Verification items for the finished model (mm, model axes). A direction names the side the tool comes from. Coordinates: 2 decimals unless noted, no trailing zeros. Write each loop counter-clockwise with the first axis right and the second up, starting at its lowest first coordinate (ties: lowest second). Pieces come first, ordered by that corner, then holes. Notation, with made-up numbers: M 12,30 L 42,30 A7 cw 42,40 Z; hole C 43.5,70 d4. An arc over 180 degrees is marked long. Answer in a Markdown table with one row per item.
from build123d import *

# Parameters (mm, degrees)
SKETCH_1_R          = 18
EXTRUDE_1_DEPTH     = 18.5
SKETCH_2_R          = 3
EXTRUDE_2_DEPTH     = 20
SKETCH_3_R          = 11
EXTRUDE_3_DEPTH     = 2
SKETCH_4_R          = 1.5
CUT_EXTRUDE_1_DEPTH = 8
SKETCH_5_R          = 4
EXTRUDE_4_DEPTH     = 20
EXTRUDE_START       = 2
SKETCH_6_R          = 11
EXTRUDE_5_DEPTH     = 2
CUT_EXTRUDE_START   = -8
SKETCH_7_R          = 1.5
CUT_EXTRUDE_2_DEPTH = 8
CUT_EXTRUDE_START_2 = -15
CUT_EXTRUDE_3_DEPTH = 15
CUT_EXTRUDE_4_DEPTH = 15
CHAMFER_1_SIZE      = 0.3


with BuildPart() as part:
    # 草图1 → 凸台-拉伸1 (new, symmetric)
    with BuildSketch(Plane.XY):
        Circle(SKETCH_1_R)
    extrude(amount=EXTRUDE_1_DEPTH, both=True)

    # 草图2 → 凸台-拉伸2 (add)
    with BuildSketch(Plane.XY.offset(18.5)):
        Circle(SKETCH_2_R)
    extrude(amount=EXTRUDE_2_DEPTH)

    # 草图3 → 凸台-拉伸3 (add)
    with BuildSketch(Plane.XY.offset(18.5)):
        Circle(SKETCH_3_R)
    extrude(amount=EXTRUDE_3_DEPTH)

    # 草图4 → 切除-拉伸1 (cut)
    with BuildSketch(Plane.XY.offset(18.5)):
        with Locations((-9.899494937, 9.899494937)):
            Circle(SKETCH_4_R)
        with Locations((9.899494937, 9.899494937)):
            Circle(SKETCH_4_R)
        with Locations((9.899494937, -9.899494937)):
            Circle(SKETCH_4_R)
        with Locations((-9.899494937, -9.899494937)):
            Circle(SKETCH_4_R)
    extrude(amount=-CUT_EXTRUDE_1_DEPTH, mode=Mode.SUBTRACT)

    # 草图5 → 凸台-拉伸4 (add)
    with BuildSketch(Plane(origin=(0, 0, -18.5), x_dir=(-1, 0, 0), z_dir=(0, 0, -1))):
        Circle(SKETCH_5_R)
    extrude(amount=EXTRUDE_4_DEPTH)

    # 草图6 → 凸台-拉伸5 (add)
    with BuildSketch(Plane(origin=(0, 0, -18.5), x_dir=(-1, 0, 0), z_dir=(0, 0, -1)).offset(EXTRUDE_START)):
        with Locations(Location((0, 0, 0), (0, 0, 180))):
            Circle(SKETCH_6_R)
    extrude(amount=-EXTRUDE_5_DEPTH)

    # 草图7 → 切除-拉伸2 (cut)
    with BuildSketch(Plane(origin=(0, 0, -18.5), x_dir=(-1, 0, 0), z_dir=(0, 0, -1)).offset(CUT_EXTRUDE_START)):
        with Locations(Location((-9.899494937, 9.899494937, 0), (0, 0, 180))):
            Circle(SKETCH_7_R)
        with Locations(Location((9.899494937, 9.899494937, 0), (0, 0, 180))):
            Circle(SKETCH_7_R)
        with Locations(Location((9.899494937, -9.899494937, 0), (0, 0, 180))):
            Circle(SKETCH_7_R)
        with Locations(Location((-9.899494937, -9.899494937, 0), (0, 0, 180))):
            Circle(SKETCH_7_R)
    extrude(amount=CUT_EXTRUDE_2_DEPTH, mode=Mode.SUBTRACT)

    # 草图8 → 切除-拉伸3 (cut)
    with BuildSketch(Plane.XY.offset(38.5).offset(CUT_EXTRUDE_START_2)):
        with BuildLine():
            Line((-2, 2.236067977), (-2, -2.236067977))
            ThreePointArc((-2, -2.236067977), (-3, 0), (-2, 2.236067977))
        make_face()
    extrude(amount=CUT_EXTRUDE_3_DEPTH, mode=Mode.SUBTRACT)

    # 草图9 → 切除-拉伸4 (cut)
    with BuildSketch(Plane(origin=(0, 0, -38.5), x_dir=(-1, 0, 0), z_dir=(0, 0, -1)).offset(CUT_EXTRUDE_START_2)):
        with BuildLine():
            Line((-3, 2.645751311), (-3, -2.645751311))
            ThreePointArc((-3, -2.645751311), (-4, 0), (-3, 2.645751311))
        make_face()
    extrude(amount=CUT_EXTRUDE_4_DEPTH, mode=Mode.SUBTRACT)

    # 倒角1
    chamfer_1_edges = [part.edges().sort_by_distance(p)[0] for p in [
        (1.224744871, -2.738612788, 38.5),
        (-1.414213562, -3.741657387, -38.5),
    ]]
    chamfer(chamfer_1_edges, length=CHAMFER_1_SIZE)


solid = part.part
1) Tool access check on faces 1 (the face through (-3.815, 1.201, -29.226)), 2 (the face through (8.79, -8.89, 14.56)), 3 (the face through (0, 0, -38.5)). Record the directions out of +Z, -Z, +X, -X, +Y, -Y that give a thin tool (end or side, any length) a straight path to the whole face; none if there is none.
Response values:
| item | result |
|---|---|
| face 1 | -Z |
| face 2 | +Z |
| face 3 | -Z, +X, -X, +Y, -Y |
2) Sectioned sample at A-A (y = 0). Record the cut outline in (x, z), then the cut area to 3 significant figures.
Response values:
| item | result |
|---|---|
| outline | M -18,-18.5 L -11,-18.5 L -11,-20.5 L -4,-20.5 L -4,-38.2 L -3.7,-38.5 L 3,-38.5 L 3,-23.5 L 4,-23.5 L 4,-20.5 L 11,-20.5 L 11,-18.5 L 18,-18.5 L 18,18.5 L 11,18.5 L 11,20.5 L 3,20.5 L 3,38.2 L 2.7,38.5 L -2,38.5 L -2,23.5 L -3,23.5 L -3,20.5 L -11,20.5 L -11,18.5 L -18,18.5 Z |
| area | 1,640 mm² |
3) Depth check by flat-ended pin: pin 1 (2.5 mm diameter, centred on x = -10, y = -10.5, fed in from +Z); pin 2 (11 mm diameter, centred on x = -6, y = -8.5, fed in from -Z); pin 3 (1.6 mm diameter, centred on y = -1, z = -27.5, fed in from +X). Enter the tip coordinate at first touch or a pass-through.
Response values:
| item | result |
|---|---|
| pin 1 | stops at z = 18.5 |
| pin 2 | stops at z = -20.5 |
| pin 3 | stops at x = 3 |
4) Sectioned sample at C-C (z = -5). Record the cut outline in (x, y), then the cut area to 3 significant figures.
Response values:
| item | result |
|---|---|
| outline | C 0,0 d36 |
| area | 1,020 mm² |
5) Sectioned sample at B-B (x = 0). Record the cut outline in (y, z), then the cut area to 3 significant figures.
Response values:
| item | result |
|---|---|
| outline | M -18,-18.5 L -11,-18.5 L -11,-20.5 L -4,-20.5 L -4,-38.2 L -3.7,-38.5 L 3.7,-38.5 L 4,-38.2 L 4,-20.5 L 11,-20.5 L 11,-18.5 L 18,-18.5 L 18,18.5 L 11,18.5 L 11,20.5 L 3,20.5 L 3,38.2 L 2.7,38.5 L -2.7,38.5 L -3,38.2 L -3,20.5 L -11,20.5 L -11,18.5 L -18,18.5 Z |
| area | 1,670 mm² |
6) Release check for a two-part mould opening along X. For faces 4 (the face through (-2.343, 17.847, 0.259)), 5 (the face through (-2, 0, 31)), 6 (the face through (-10, 10, 10.5)) record: +X half, -X half, draft (parallel to the pull), parting line (faces both ways), or undercut.
Response values:
| item | result |
|---|---|
| face 4 | parting line |
| face 5 | -X half |
| face 6 | undercut |
7) Thickness scan on L1, parallel to Z at x = 11, y = 14; L2, parallel to Z at x = -5.5, y = 9; L3, parallel to Y at x = -3, z = -28. Record the ranges inside material, lowest first. Write a range as [from, to].
Response values:
| item | result |
|---|---|
| L1 | z = [-18.5, 18.5] |
| L2 | z = [-20.5, 20.5] |
| L3 | y = [-2.65, 2.65] |
8) Sectioned sample at D-D (y = 5.5). Record the cut outline in (x, z), then the cut area to 3 significant figures.
Response values:
| item | result |
|---|---|
| outline | M -17.14,-18.5 L -9.53,-18.5 L -9.53,-20.5 L 9.53,-20.5 L 9.53,-18.5 L 17.14,-18.5 L 17.14,18.5 L 9.53,18.5 L 9.53,20.5 L -9.53,20.5 L -9.53,18.5 L -17.14,18.5 Z |
| area | 1,340 mm² |
